Part model, mm, in its own coordinate system. A direction names the side the tool comes from. Coordinates: 2 decimals unless noted, no trailing zeros. Order: outer loops, then holes, each group sorted by start corner. A loop starts at its lowest first (then second) coordinate and runs counter-clockwise, first axis right, second up.
1) Cut at B-B (x = 3.75). List the corners of the cut face in (y, z), and give its area (3 significant figures).
2) Wall check: L1, parallel to X at y = 0, z = 5; L2, parallel to Y at x = 0, z = 6.5; L3, parallel to Y at x = 10, z = 3.75. Give the ranges that are in metal, low to high.
3) Mould opens along Y. For faces 5 (the cylindrical face through (-11.687, 1.953, 4.93)), 6 (the conical face through (-11.301, 7.02, 0.286)), 7 (the cylindrical face through (-9.44, -6.65, 4.93)) say: +Y half, -Y half, draft (parallel to the pull), parting line (faces both ways), or undercut.
4) Pin check, flat tips, straight feed: pin 1 Ø1.8 at (x, z) = (-0.5, 7) entering from -Y; pin 2 Ø6 at (y, z) = (-4, 5.5) entering from +X; pin 3 Ø1.2 at (y, z) = (4.5, 7.5) entering from -X; pin 4 Ø0.8 at (y, z) = (5.5, 6) entering from +X. Stop position of each tip, or through.
5) Tool access for faces 1 (the flat face through (-3, 5, 5)), 2 (the cylindrical face through (1.455, -11.261, 4.93)), 3 (the cylindrical face through (-9.38, 7.6, 4.93)), 4 (the cylindrical face through (-10.894, 5.089, 4.93)): list every direction of +Z, -Z, +X, -X, +Y, -Y with a clear straight run to the whole face (end or side of a thin tool).
6) Cut at A-A (x = 0). List the corners of the cut face in (y, z), and give its area (3 significant figures).
```python
from build123d import *

# Parameters (mm, degrees)
BOSS_EXTRUDE1_DEPTH          = 10
CHAMFER1_SIZE                = 0.75
CIRPATTERN1_COUNT            = 12
CHAMFER1_OF_CIRPATTERN1_SIZE = 0.75
CUT_EXTRUDE2_DEPTH           = 10


with BuildPart() as part:
    # Sketch1 → Boss-Extrude1 (new body)
    with BuildSketch(Plane.XY):
        with BuildLine():
            ThreePointArc((-2.07, 9.271736623), (0, -9.5), (2.07, 9.271736623))
            ThreePointArc((2.07, 9.271736623), (1.625653209, 11.72726856), (0.57, 13.988391616))
            ThreePointArc((0.57, 13.988391616), (0, 14), (-0.57, 13.988391616))
            ThreePointArc((-0.57, 13.988391616), (-1.625653209, 11.72726856), (-2.07, 9.271736623))
        make_face()
    boss_extrude1 = extrude(amount=BOSS_EXTRUDE1_DEPTH)

    # Chamfer1
    chamfer1_edges = [part.edges().sort_by_distance(p)[0] for p in [
        (0, 14, 10),
        (0, 14, 0),
    ]]
    chamfer(chamfer1_edges, length=CHAMFER1_SIZE)

    # CirPattern1: Boss-Extrude1 ×12 about axis
    cirpattern1_axis = Axis((0, 0.479093936, 0), (0, 0, 1))
    for i in range(1, CIRPATTERN1_COUNT):
        add(boss_extrude1.rotate(cirpattern1_axis, i * 360 / CIRPATTERN1_COUNT))

    # Chamfer1 of CirPattern1
    chamfer1_of_cirpattern1_edges = [part.edges().sort_by_distance(p)[0] for p in [
        (-6.760453032, 12.18854207, 10),
        (-6.760453032, 12.18854207, 0),
        (-11.709448133, 7.239546968, 10),
        (-11.709448133, 7.239546968, 0),
        (-13.520906064, 0.479093936, 10),
        (-13.520906064, 0.479093936, 0),
        (-11.709448133, -6.281359096, 10),
        (-11.709448133, -6.281359096, 0),
        (-6.760453032, -11.230354197, 10),
        (-6.760453032, -11.230354197, 0),
        (0, -13.041812128, 10),
        (0, -13.041812128, 0),
        (6.760453032, -11.230354197, 10),
        (6.760453032, -11.230354197, 0),
        (11.709448133, -6.281359096, 10),
        (11.709448133, -6.281359096, 0),
        (13.520906064, 0.479093936, 10),
        (13.520906064, 0.479093936, 0),
        (11.709448133, 7.239546968, 10),
        (11.709448133, 7.239546968, 0),
        (6.760453032, 12.18854207, 10),
        (6.760453032, 12.18854207, 0),
    ]]
    chamfer(chamfer1_of_cirpattern1_edges, length=CHAMFER1_OF_CIRPATTERN1_SIZE)

    # Sketch3 → Cut-Extrude2 (cut)
    with BuildSketch(Plane.XY.offset(10)):
        with BuildLine():
            Line((-3, 4.25), (-3, 5.766281297))
            ThreePointArc((-3, 5.766281297), (-3.372684391, -5.556527693), (6.5, 0))
            ThreePointArc((6.5, 0), (5.556527693, 3.372684391), (3, 5.766281297))
            Line((3, 5.766281297), (3, 4.25))
            Line((3, 4.25), (-3, 4.25))
        make_face()
    extrude(amount=-CUT_EXTRUDE2_DEPTH, mode=Mode.SUBTRACT)


solid = part.part
```
Geometry check:
1. outline: (-9.62, 0) - (-5.31, 0) - (-5.31, 10) - (-9.62, 10) - close; (5.31, 0) - (10.58, 0) - (10.58, 10) - (5.31, 10) - close
1. area: 95.8 mm2
2. L1: x = -13.51 to -6.5, 6.5 to 13.51
2. L2: y = -13.04 to -6.5, 4.25 to 14
2. L3: y = -6.73 to -3.18, -1.45 to 2.41, 4.14 to 7.68
3. face 5: undercut
3. face 6: +Y half
3. face 7: -Y half
4. pin 1: stops at y = -13.04
4. pin 2: stops at x = 11.98
4. pin 3: stops at x = -10.9
4. pin 4: stops at x = 11.49
5. face 1: +Z, -Z
5. face 2: +Z, -Z, -Y
5. face 3: +Z, -Z, +Y
5. face 4: +Z, -Z, -X
6. outline: (-13.04, 0.75) - (-12.29, 0) - (-6.5, 0) - (-6.5, 10) - (-12.29, 10) - (-13.04, 9.25) - close; (4.25, 0) - (13.25, 0) - (14, 0.75) - (14, 9.25) - (13.25, 10) - (4.25, 10) - close
6. area: 162 mm2
